from build123d import *

# Parameters (mm, degrees)
SKETCH1_R           = 150
BOSS_EXTRUDE1_DEPTH = 30


with BuildPart() as part:
    # Sketch1 → Boss-Extrude1 (new body)
    with BuildSketch(Plane.XY):
        Circle(SKETCH1_R)
        with BuildLine():
            Line((-50, -10), (-50, 10))
            Line((-50, 10), (-28.284271247, 10))
            ThreePointArc((-28.284271247, 10), (0, 30), (28.284271247, 10))
            Line((28.284271247, 10), (50, 10))
            Line((50, 10), (50, -10))
            Line((50, -10), (28.284271247, -10))
            ThreePointArc((28.284271247, -10), (0, -30), (-28.284271247, -10))
            Line((-28.284271247, -10), (-50, -10))
        make_face(mode=Mode.SUBTRACT)
    extrude(amount=BOSS_EXTRUDE1_DEPTH)


solid = part.part
Read the model definition and answer for the solid it produces. Units are mm, in the model's axes. A direction names the side the tool comes from. Give positions to 0.01 mm unless a question says otherwise; leave off trailing zeros. Write each loop counter-clockwise with the first axis right and the second up, starting at its lowest first coordinate (ties: lowest second). Pieces come first, ordered by that corner, then holes. Notation, with made-up numbers: (56.25, -12.5) - (109.25, -12.5) arc R14 ccw to (109.25, -1.5) - close; hole circle Ø9 at (-21, 16). An arc over 180 degrees is marked (long way). Use CSV: the item, a comma, the result in double quotes. Start each with the question number.
(1) Determine the mould class of faces 1 (the cylindrical face through (-0.517, 29.996, 14.79)), 2 (the flat face through (-2, -31, 0)), 3 (the cylindrical face through (-19.527, 148.724, 14.79)) for opening direction X: +X half, -X half, draft (parallel to the pull), parting line (faces both ways), or undercut.
(2) Given P1, Ø17.5, axis at x = 35, z = 9.5, coming from the -Y side; P2, Ø6.5, axis at x = -34.5, z = 19.5, coming from the +Y side; P3, Ø4, axis at x = -81, z = 18.5, coming from the +Y side, each flat-ended and moving along its own axis, determine where each tip first touches the part or whether it passes through.
(3) For faces 4 (the flat face through (-50, 0, 15)), 5 (the flat face through (-2, -31, 30)), determine the directions among +Z, -Z, +X, -X, +Y, -Y from which every point of the face is accessible in a straight line to the end or side of a thin tool.
(4) Find section D-D (y = 86). Give the vertices of the cut face in (x, z).
(5) Find section C-C (z = 17). Give the vertices of the cut face in (x, y), plus the area to 3 significant figures.
(6) Find section B-B (y = 0). Give the vertices of the cut face in (x, z).
(7) Find section A-A (x = 0). Give the vertices of the cut face in (y, z).
(8) Consider line 1 along Y through (x, z) = (-20, 2.5); line 2 along Y through (x, z) = (45, 20.5); line 3 along Y through (x, z) = (60, 28.5). Determine where each line is inside the solid, lowest interval first.
Findings below:
1,face 1,"undercut"
1,face 2,"draft"
1,face 3,"parting line"
2,P1,"y = -147.69"
2,P2,"y = 146.71"
2,P3,"y = 127.51"
3,face 4,"+Z, -Z"
3,face 5,"+Z, +X, -X, +Y, -Y"
4,outline,"(-122.9, 0) - (122.9, 0) - (122.9, 30) - (-122.9, 30) - close"
5,outline,"circle Ø300 at (0, 0); hole (-50, -10) - (-28.28, -10) arc R30 ccw to (28.28, -10) - (50, -10) - (50, 10) - (28.28, 10) arc R30 ccw to (-28.28, 10) - (-50, 10) - close"
5,area,"67,000 mm2"
6,outline,"(-150, 0) - (-50, 0) - (-50, 30) - (-150, 30) - close; (50, 0) - (150, 0) - (150, 30) - (50, 30) - close"
7,outline,"(-150, 0) - (-30, 0) - (-30, 30) - (-150, 30) - close; (30, 0) - (150, 0) - (150, 30) - (30, 30) - close"
8,line 1,"-148.66 to -22.36, 22.36 to 148.66"
8,line 2,"-143.09 to -10, 10 to 143.09"
8,line 3,"-137.48 to 137.48"
